For this review, take the finished solid that the model builds, in its own axes (mm). Round coordinates to 2 decimals unless told otherwise and drop trailing zeros. Write each loop counter-clockwise with the first axis right and the second up, starting at its lowest first coordinate (ties: lowest second). Pieces come first, ordered by that corner, then holes. Notation, with made-up numbers: M -38,82.5 L 7,82.5 A32 ccw 7,121.5 Z; hole C -9.5,9 d8. An arc over 180 degrees is marked long. Use one line per item in the form item = value. Start each with the question number.
Item 1: Add section A-A (y = 1.8). State the section outline as (x, z) points, and give its area (3 significant figures).
Item 2: Add section B-B (z = 121.75). State the section outline as (x, y) points, and give its area (3 significant figures).
Item 3: Add section C-C (z = 216.1). State the section outline as (x, y) points.
Item 4: For line 1 (X direction, y = 1.45, z = -2); line 2 (Z direction, x = 15, y = 1.25); line 3 (Z direction, x = 17.5, y = 1.45), list the stretches that pass through material, from the lowest coordinate up. Write a range as [from, to].
Item 5: Draft analysis for pull direction Z (two halves, no side actions). For faces 1 (the flat face through (22, 0, 3)), 2 (the cylindrical face through (15.78, 1.27, -118.3)), 3 (the cylindrical face through (18.021, 1.268, -209.634)), state which applies: released by +Z, released by -Z, zero draft, split by the parting line, or undercut.
from build123d import *

# Parameters (mm, degrees)
BOSS_EXTRUDE1_DEPTH = 226.1
SKETCH2_R           = 4
SKETCH2_R_2         = 6
CUT_EXTRUDE1_DEPTH  = 229.095287106


with BuildPart() as part:
    # Sketch1 → Boss-Extrude1 (new, symmetric)
    with BuildSketch(Plane.XY):
        Polygon((0, 0), (0, 2.5), (2.5, 2.5), (30, 2.5), (30, 0), align=None)
    extrude(amount=BOSS_EXTRUDE1_DEPTH, both=True)

    # Sketch2 → Cut-Extrude1 (cut, through all)
    with BuildSketch(Plane(origin=(0, 2.5, 0), x_dir=(1, 0, 0), z_dir=(0, 1, 0))):
        with Locations(Location((17.5, 213.6, 0), (0, 0, 180))):
            Circle(SKETCH2_R)
        with Locations((17.5, -216.1)):
            Circle(SKETCH2_R)
        with Locations(Location((15, -121.75, 0), (0, 0, 180))):
            Circle(SKETCH2_R_2)
        with Locations(Location((15, 124.25, 0), (0, 0, 180))):
            Circle(SKETCH2_R_2)
        with Locations(Location((15, 1.25, 0), (0, 0, 180))):
            Circle(SKETCH2_R_2)
    extrude(amount=-CUT_EXTRUDE1_DEPTH, mode=Mode.SUBTRACT)


solid = part.part
Calculated:
q1.outline = M 0,-226.1 L 30,-226.1 L 30,226.1 L 0,226.1 Z; hole C 15,-124.25 d12; hole C 15,-1.25 d12; hole C 15,121.75 d12; hole C 17.5,-213.6 d8; hole C 17.5,216.1 d8
q1.area = 13,100 mm^2
q2.outline = M 0,0 L 9,0 L 9,2.5 L 0,2.5 Z; M 21,0 L 30,0 L 30,2.5 L 21,2.5 Z
q2.area = 45.0 mm^2
q3.outline = M 0,0 L 13.5,0 L 13.5,2.5 L 0,2.5 Z; M 21.5,0 L 30,0 L 30,2.5 L 21.5,2.5 Z
q4.line_1 = [0, 9.05], [20.95, 30]
q4.line_2 = [-226.1, -216.72], [-210.48, -130.25], [-118.25, -7.25], [4.75, 115.75], [127.75, 212.98], [219.22, 226.1]
q4.line_3 = [-226.1, -217.6], [-209.6, -129.7], [-118.8, -6.7], [4.2, 116.3], [127.2, 212.1], [220.1, 226.1]
q5.face_1 = zero draft
q5.face_2 = undercut
q5.face_3 = undercut
